Geometry check sheet. Reference: the model listing, model coordinates, mm. Face numbers are marked on the shaded views. A direction names the side the tool comes from. Round coordinates to 2 decimals unless told otherwise and drop trailing zeros. Loops run counter-clockwise (first coordinate to the right, second up) from the corner with the lowest first, then second, coordinate; pieces in that order, holes last.
```python
from build123d import *

# Parameters (mm, degrees)
F0_R     = 5
F1_DEPTH = 15
F3_D     = 5.5
F4_R     = 2
F5_DEPTH = 5
F6_D     = 4.4
F6_DEPTH = 8
F6_TIP   = 1.3218933619
F7_R     = 3
F8_DEPTH = 25


with BuildPart() as f1:
    # F0 (on Front) → F1 (new body)
    with BuildSketch(Plane.XZ):
        with BuildLine():
            Line((0, 44.4), (0, 0))
            Line((0, 0), (16, 0))
            Line((16, 0), (16, 28.1794662359))
            Line((16, 28.1794662359), (6.183998533, 34.1947196713))
            ThreePointArc((6.183998533, 34.1947196713), (5.2289956624, 35.9), (6.183998533, 37.6052803287))
            Line((6.183998533, 37.6052803287), (18.9071712183, 42.2361364716))
            Line((18.9071712183, 42.2361364716), (16, 50.2235237483))
            Line((16, 50.2235237483), (0, 44.4))
        make_face()
        with Locations((7.2, 25)):
            Circle(F0_R, mode=Mode.SUBTRACT)
    extrude(amount=F1_DEPTH)

    # F3 (through all)
    with Locations(Plane(origin=(-14.269884935, 0, 39.2061866372), x_dir=(0.9396926208, 0, 0.3420201433), z_dir=(-0.3420201433, 0, 0.9396926208))):
        with Locations((25.9125387233, -7.5)):
            Hole(F3_D / 2)

    # F4 (on face) → F5 (cut)
    with BuildSketch(Plane(origin=(0, 0, 0), x_dir=(1, 0, 0), z_dir=(0, 0, -1))):
        with Locations((3.5, 7.5)):
            Circle(F4_R)
    extrude(amount=-F5_DEPTH, mode=Mode.SUBTRACT)

    # F6
    with Locations(Plane(origin=(0, 0, 0), x_dir=(1, 0, 0), z_dir=(0, 0, -1))):
        with Locations((8, 12.5), (8, 2.5)):
            Hole(F6_D / 2, depth=F6_DEPTH)
            with Locations((0, 0, -(F6_DEPTH + F6_TIP / 2))):  # 118° drill point
                Cone(0, F6_D / 2, F6_TIP, mode=Mode.SUBTRACT)

    # F7 (on face) → F8 (cut)
    with BuildSketch(Plane(origin=(-11.3627137168, 0, 31.2187993606), x_dir=(0.9396926208, 0, 0.3420201433), z_dir=(0.3420201433, 0, -0.9396926208))):
        with Locations((25.9125387233, 7.5)):
            Circle(F7_R)
    extrude(amount=F8_DEPTH, mode=Mode.SUBTRACT)


solid = f1.part
```
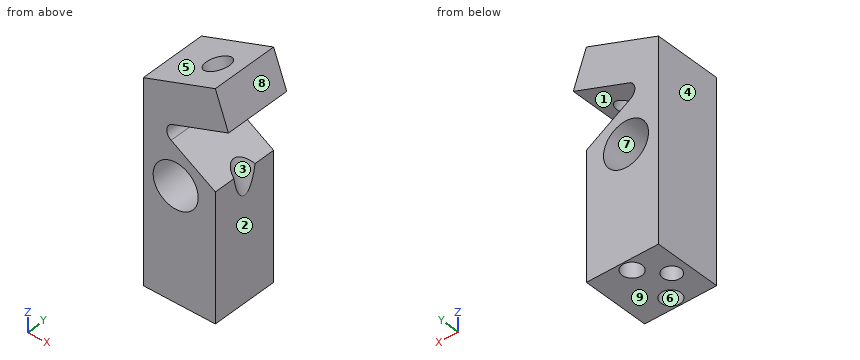
1) Gauge pin test, flat ends, axial feed: pin 1 (1.5 mm diameter, centred on x = 7.5, y = -12, fed in from -Z); pin 2 (1 mm diameter, centred on x = 5.5, y = -10, fed in from +Z); pin 3 (8 mm diameter, centred on y = -12, z = 15.5, fed in from +X). Record the tip position at first contact, or that the pin passes through.
Report:
pin 1: stops at z = 8.45
pin 2: stops at z = 46.58
pin 3: stops at x = 16
2) Sectioned sample at A-A, the plane y = -7. Record the cut outline in (x, z).
Report:
outline: (0, 0) - (1.56, 0) - (1.56, 5) - (5.44, 5) - (5.44, 0) - (16, 0) - (16, 23.15) - (13.65, 29.62) - (6.18, 34.19) arc R2 cw to (6.18, 37.61) - (10.45, 39.16) - (7.54, 47.14) - (0, 44.4) - close; (12.62, 48.99) - (15.53, 41.01) - (18.91, 42.24) - (16, 50.22) - close; hole circle Ø10 at (7.2, 25)
3) Access from +Z, -Z, +X, -X, +Y, -Y to the whole of each face (thin tool, end or side, straight path). Record for the marked faces 1, 2, 3, 4 and 5.
Report:
face 1: +X, +Y, -Y
face 2: -Z, +X, +Y, -Y
face 3: +X
face 4: +Z, -Z, -X, +Y, -Y
face 5: +Z, -X, +Y, -Y
4) Scan lines: line 1 along Y through (x, z) = (8, 6.5); line 2 along Z through (x, y) = (9.75, -1.75); line 3 along X through (y, z) = (-12.5, 5). Record each from-to range of solid material in increasing order.
Report:
line 1: y = -15 to -14.7, -10.3 to -4.7, -0.3 to 0
line 2: z = 8.18 to 20.7, 29.3 to 32.01, 38.9 to 47.95
line 3: x = 0 to 5.8, 10.2 to 16
5) Sectioned sample at C-C, the plane x = 7. State how many separate pieces and enclosed holes the cut face has, then the cut area to 3 significant figures.
Report:
separate pieces: 3
enclosed holes: 0
area: 425 mm2
6) Sectioned sample at D-D, the plane z = 32.5. Record the cut outline in (x, y), then the cut area to 3 significant figures.
Report:
outline: (0, -15) - (8.95, -15) - (8.95, 0) - (0, 0) - close
area: 134 mm2
7) Mould release check, pull along X, two halves, no side actions. Record for the marked faces 6, 7, 8 and 9: +X half, -X half, draft (parallel to the pull), parting line (faces both ways), or undercut.
Report:
face 6: undercut
face 7: undercut
face 8: +X half
face 9: draft
8) Sectioned sample at B-B, the plane z = 4.5. Record the cut outline in (x, y).
Report:
outline: (0, -15) - (16, -15) - (16, 0) - (0, 0) - close; hole circle Ø4 at (3.5, -7.5); hole circle Ø4.4 at (8, -12.5); hole circle Ø4.4 at (8, -2.5)
